```python
from build123d import *

# Parameters (mm, degrees)
F1_DEPTH = 1247
F2_W     = 2
F2_H     = 157
F3_DEPTH = 36.5
F4_W     = 2
F4_H     = 157
F5_DEPTH = 36.5
F6_R     = 2
F7_DEPTH = 17.182757


with BuildPart() as f1:
    # F0 (on Right) → F1 (new body)
    with BuildSketch(Plane.YZ):
        with BuildLine():
            Line((-0.923239, 122.649228), (-2.923239, 122.649228))
            Line((-2.923239, 122.649228), (-2.923239, -34.350772))
            ThreePointArc((-2.923239, -34.350772), (-1.643968, -36.808228), (1.102821, -37.16985))
            Line((1.102821, -37.16985), (14.258518, -32.381568))
            Line((14.258518, -32.381568), (13.574478, -30.502182))
            Line((13.574478, -30.502182), (0.418781, -35.290464))
            ThreePointArc((0.418781, -35.290464), (-0.496816, -35.169924), (-0.923239, -34.350772))
            Line((-0.923239, -34.350772), (-0.923239, 122.649228))
        make_face()
    extrude(amount=F1_DEPTH)

    # F2 (on face) → F3 (join)
    with BuildSketch(Plane.YZ.offset(1247)):
        with Locations((-1.923239, 44.149228)):
            Rectangle(F2_W, F2_H)
    extrude(amount=F3_DEPTH)

    # F4 (on face) → F5 (join)
    with BuildSketch(Plane(origin=(0, 0, 0), x_dir=(0, -1, 0), z_dir=(-1, 0, 0))):
        with Locations((1.923239, 44.149228)):
            Rectangle(F4_W, F4_H)
    extrude(amount=F5_DEPTH)

    # F6 (on face) → F7 (cut, through all)
    with BuildSketch(Plane.XZ.offset(2.923239)):
        with Locations((-21.5, 107.649228)):
            Circle(F6_R)
        with Locations((-21.5, -19.350772)):
            Circle(F6_R)
        with Locations((1268.5, 107.649228)):
            Circle(F6_R)
        with Locations((1268.5, -19.350772)):
            Circle(F6_R)
    extrude(amount=-F7_DEPTH, mode=Mode.SUBTRACT)


solid = f1.part
```
Can you work these out from the model? Positions are in its coordinate system, mm. Round coordinates to 2 decimals unless told otherwise and drop trailing zeros. Loops run counter-clockwise (first coordinate to the right, second up) from the corner with the lowest first, then second, coordinate; pieces in that order, holes last. Notation, with made-up numbers: (27.25, 74.25) -> (70.25, 74.25) arc R22 cw to (70.25, 113.25) -> close; hole circle Ø5 at (-18, 87.25). An arc over 180 degrees is marked (long way). One line per item, written item: value. Start each with the question number.
1. For pin 1 (2.5 mm diameter, centred on x = -21.5, z = -19.35, fed in from -Y); pin 2 (2 mm diameter, centred on y = 5, z = -35.5, fed in from -X); pin 3 (0.6 mm diameter, centred on x = 1260.5, y = -2, fed in from -Z); pin 4 (1.5 mm diameter, centred on x = 1056, y = 4, fed in from +Z), each with a flat end and sliding along its axis, tell me the tip position at first contact or that it passes through.
2. If we section it at B-B, the plane z = 14.5: Write out the boundary of the cut face in (x, y), then the cut area to 3 significant figures.
3. If we section it at C-C, the plane y = 4.5: Write out the boundary of the cut face in (x, z).
4. If I drill on probe 1 along Y at (x, z) = (577.5, 63); probe 2 along Z at (x, y) = (555, 0.75); probe 3 along Z at (x, y) = (571, 3.5), over which ranges is the centre line in solid material (lowest first)?
5. If we section it at A-A, the plane x = 678: Write out the boundary of the cut face in (y, z).
Calculated:
1. pin 1: passes through
1. pin 2: stops at x = 0
1. pin 3: stops at z = -34.35
1. pin 4: stops at z = -33.71
2. outline: (-36.5, -2.92) -> (1283.5, -2.92) -> (1283.5, -0.92) -> (-36.5, -0.92) -> close
2. area: 2,640 mm²
3. outline: (0, -35.93) -> (1247, -35.93) -> (1247, -33.81) -> (0, -33.81) -> close
4. probe 1: y = -2.92 to -0.92
4. probe 2: z = -37.27 to -35.17
4. probe 3: z = -36.3 to -34.17
5. outline: (-2.92, -34.35) arc R3 ccw to (1.1, -37.17) -> (14.26, -32.38) -> (13.57, -30.5) -> (0.42, -35.29) arc R1 cw to (-0.92, -34.35) -> (-0.92, 122.65) -> (-2.92, 122.65) -> close
